from build123d import *

# Parameters (mm, degrees)
SKETCH1_W           = 635.3556
SKETCH1_H           = 266.7
BOSS_EXTRUDE1_DEPTH = 1.143
SKETCH2_W           = 254
SKETCH2_H           = 2.7305
BOSS_EXTRUDE2_DEPTH = 3.175
CUT_EXTRUDE1_DEPTH  = 10
LPATTERN1_COUNT     = 5
LPATTERN1_PITCH     = 140.97


with BuildPart() as part:
    # Sketch1 → Boss-Extrude1 (new, symmetric)
    with BuildSketch(Plane(origin=(0, 0, 0), x_dir=(1, 0, 0), z_dir=(0, 1, 0))):
        Rectangle(SKETCH1_W, SKETCH1_H)
    extrude(amount=BOSS_EXTRUDE1_DEPTH, both=True)

    # Sketch2 → Boss-Extrude2 (add)
    with BuildSketch(Plane(origin=(0, 0, -133.35), x_dir=(-1, 0, 0), z_dir=(0, 0, -1))):
        with Locations((-157.8229, 0.22225)):
            Rectangle(SKETCH2_W, SKETCH2_H)
        with Locations((157.8229, 0.22225)):
            Rectangle(SKETCH2_W, SKETCH2_H)
    extrude(amount=BOSS_EXTRUDE2_DEPTH)

    # Sketch3 → Cut-Extrude1 (cut, symmetric)
    with BuildSketch(Plane(origin=(0, 1.143, 0), x_dir=(1, 0, 0), z_dir=(0, 1, 0))):
        with BuildLine():
            ThreePointArc((-275.2528, -124.714), (-274.659691232, -126.145891232), (-273.2278, -126.739))
            Line((-273.2278, -126.739), (-273.2278, -124.714))
            Line((-273.2278, -124.714), (-275.2528, -124.714))
        make_face()
        with BuildLine():
            Line((-273.2278, -124.714), (-273.2278, -126.739))
            ThreePointArc((-273.2278, -126.739), (-271.795908768, -126.145891232), (-271.2028, -124.714))
            ThreePointArc((-271.2028, -124.714), (-273.2278, -122.689), (-275.2528, -124.714))
            Line((-275.2528, -124.714), (-273.2278, -124.714))
        make_face()
    cut_extrude1 = extrude(amount=CUT_EXTRUDE1_DEPTH, both=True, mode=Mode.SUBTRACT)

    # LPattern1: Cut-Extrude1 ×5
    with Locations(*[(i * LPATTERN1_PITCH, 0, 0) for i in range(1, LPATTERN1_COUNT)]):
        add(cut_extrude1, mode=Mode.SUBTRACT)


solid = part.part
Source: CAD feature listing. Evaluate the final solid. Frame: model axes, mm. Give positions to 0.01 mm unless a question says otherwise; leave off trailing zeros. Order: outer loops, then holes, each group sorted by start corner. A loop starts at its lowest first (then second) coordinate and runs counter-clockwise, first axis right, second up. Notation, with made-up numbers: (-26, -5.5) -> (18, -5.5) arc R14 ccw to (18, 14.5) -> close; hole circle Ø3 at (50, 17.5). An arc over 180 degrees is marked (long way). Use a Markdown table: item, result.
1) Mould query, pull axis Y, two halves, no side actions, for faces 1 (the flat face through (4, -1.143, 0)), 2 (the flat face through (-4, 1.143, -2)). Classes: +Y half, -Y half, draft (parallel to the pull), parting line (faces both ways), or undercut.
Answer list:
| item | result |
|---|---|
| face 1 | -Y half |
| face 2 | +Y half |
2) Section query B-B, the plane z = 37. Return the cut outline in (x, y).
Answer list:
| item | result |
|---|---|
| outline | (-317.68, -1.14) -> (317.68, -1.14) -> (317.68, 1.14) -> (-317.68, 1.14) -> close |
3) Contact query for flat-ended pins moving along their axis: P1, Ø8, axis at x = 7, z = 43, coming from the +Y side; P2, Ø1.1, axis at x = 0.5, y = -0.5, coming from the -Z side; P3, Ø0.8, axis at y = 1, z = -135.5, coming from the -X side. Output: stop coordinate, or through.
Answer list:
| item | result |
|---|---|
| P1 | y = 1.14 |
| P2 | z = -133.35 |
| P3 | x = -284.82 |
4) Ray query, line 1 along Y through (x, z) = (-232.5, -38.5); line 2 along Z through (x, y) = (29, 0.7); line 3 along Z through (x, y) = (190, 1.4) (3 decimals). Return the intervals inside material, ascending. Write a range as [from, to].
Answer list:
| item | result |
|---|---|
| line 1 | [-1.14, 1.14] |
| line 2 | [-133.35, 133.35] |
| line 3 | [-136.525, -133.35] |
